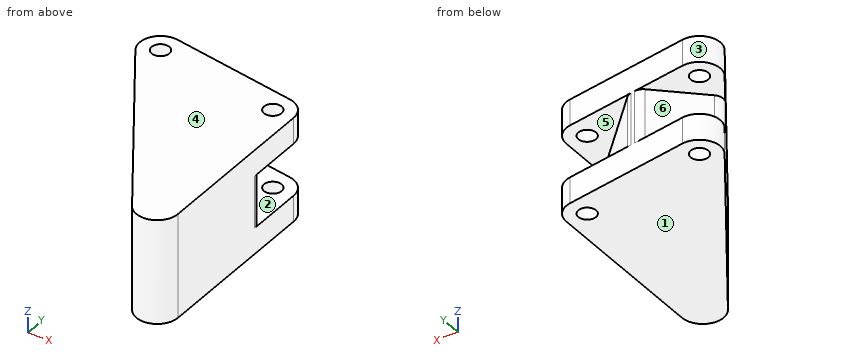
Autodesk Inventor part; units mm, degrees
ref_plane "YZ Plane" through (0, 0, 0) normal (1, 0, 0) x (0, 1, 0)
ref_plane "XZ Plane" through (0, 0, 0) normal (0, 1, 0) x (-1, 0, 0)
ref_plane "XY Plane" through (0, 0, 0) normal (0, 0, 1) x (1, 0, 0)
sketch "Sketch1" plane through (0, 0, 0) normal (0, 0, 1) x (1, 0, 0)
  line L0 (0, 0) -> (-24.2225, 3.8783) construction
  line L1 (-24.2225, 3.8783) -> (0, -32.7525) construction
  line L2 (0, -32.7525) -> (0, 0) construction
  line L3 (0.6324, 3.9497) -> (-23.5901, 7.828)
  line L4 (-27.559, 1.672) -> (-3.3365, -34.9588)
  line L5 (4, -32.7525) -> (4, 0)
  arc A0 (-23.5901, 7.828) -> (-27.559, 1.672) centre (-24.2225, 3.8783) ccw
  arc A1 (4, 0) -> (0.6324, 3.9497) centre (0, 0) ccw
  arc A2 (-3.3365, -34.9588) -> (4, -32.7525) centre (0, -32.7525) ccw
  dimension "d0" = 32.7525
  dimension "d6" = 24.531
  dimension "d14" = 43.9153
  dimension "d15" = 4
extrude "Extrusion1" add sketch "Sketch1" along normal mid plane 20
sketch "Sketch2" plane through (0, 0, 0) normal (0, 0, 1) x (1, 0, 0)
  arc A0 (-23.5901, 7.828) -> (-27.559, 1.672) centre (-24.2225, 3.8783) ccw construction
  line L0 (-3.3365, -34.9588) -> (-27.559, 1.672) construction
  arc A1 (-3.3365, -34.9588) -> (4, -32.7525) centre (0, -32.7525) ccw construction
  line L1 (4, 0) -> (4, -32.7525) construction
  arc A2 (4, 0) -> (0.6324, 3.9497) centre (0, 0) ccw construction
  line L2 (-23.5901, 7.828) -> (0.6324, 3.9497) construction
  arc A3 (4, 0) -> (0.6324, 3.9497) centre (0, 0) ccw
  line L3 (4, 0) -> (4, -10.3073)
  arc A4 (-3.3365, -34.9588) -> (4, -32.7525) centre (0, -32.7525) ccw construction
  line L4 (-3.3365, -34.9588) -> (-7.3441, -28.8984) construction
  arc A5 (-23.5901, 7.828) -> (-27.559, 1.672) centre (-24.2225, 3.8783) ccw
  line L5 (-23.5901, 7.828) -> (-14.2736, 6.3363)
  line L6 (-24.408, -3.0932) -> (-14.2736, 6.3363)
  line L7 (-11.9287, 5.9609) -> (4, -10.3073)
  line L8 (-7.3441, -28.8984) -> (4, -26.0222) construction
  line L9 (-24.408, -3.0932) -> (-27.559, 1.672)
  line L10 (-7.3441, -28.8984) -> (-24.408, -3.0932) construction
  line L11 (4, -10.3073) -> (4, -26.0222) construction
  line L12 (4, -26.0222) -> (4, -32.7525) construction
  line L13 (-11.9287, 5.9609) -> (0.6324, 3.9497)
  line L14 (-14.2736, 6.3363) -> (-11.9287, 5.9609) construction
extrude "Extrusion2" cut sketch "Sketch2" along normal mid plane 10
fillet "Fillet1" radius 2 4 edges at (4, -10.3073, 0) (-11.9287, 5.9609, 0) (-24.408, -3.0932, 0) (-14.2736, 6.3363, 0)
sketch "Sketch3" plane through (0, 0, 10) normal (0, 0, 1) x (1, 0, 0)
  arc A0 (-23.5901, 7.828) -> (-27.559, 1.672) centre (-24.2225, 3.8783) ccw construction
  arc A1 (-3.3365, -34.9588) -> (4, -32.7525) centre (0, -32.7525) ccw construction
  arc A2 (4, 0) -> (0.6324, 3.9497) centre (0, 0) ccw construction
hole "Hole1" at (-24.2225, 3.8783, 10) at (0, 0, 10) direction (0, 0, -1) diameter 3.4 end through all
equation "\"d0\" = LengthI"
equation "\"d6\" = LengthG"
equation "\"d14\" = LengthH"
properties part number "GHI"
Verification items for the finished model (mm, model axes). Face numbers are marked on the shaded views. A direction names the side the tool comes from. Round coordinates to 2 decimals unless told otherwise and drop trailing zeros. Order: outer loops, then holes, each group sorted by start corner. A loop starts at its lowest first (then second) coordinate and runs counter-clockwise, first axis right, second up.
1) Material ranges on line 1 (X direction, y = 1, z = 6.75); line 2 (Y direction, x = -24, z = 8.5); line 3 (X direction, y = 0, z = 8.9), recorded low to high.
Geometry says:
line 1: x = -27.11 to -1.37, 1.37 to 3.87
line 2: y = -3.71 to 2.19, 5.56 to 7.87
line 3: x = -26.45 to -1.7, 1.7 to 4
2) Depth check by flat-ended pin: pin 1 (2 mm diameter, centred on x = -20.5, z = 5, fed in from -Y); pin 2 (10 mm diameter, centred on y = -29.5, z = 2.5, fed in from -X); pin 3 (8 mm diameter, centred on y = -10, z = 2.5, fed in from -X). Enter the tip coordinate at first touch or a pass-through.
Geometry says:
pin 1: stops at y = -10.52
pin 2: stops at x = -10.25
pin 3: stops at x = -22.49
3) Draft check along Z on the marked faces 1, 2 and 3. Enter one of: +Z half, -Z half, draft (parallel to the pull), parting line (faces both ways), or undercut.
Geometry says:
face 1: -Z half
face 2: undercut
face 3: draft
4) Cross-section at B-B, the plane x = -21.5. Record the cut outline in (y, z).
Geometry says:
outline: (-7.49, -10) - (7.49, -10) - (7.49, -5) - (-0.39, -5) - (-0.39, 5) - (7.49, 5) - (7.49, 10) - (-7.49, 10) - close
5) Cross-section at D-D, the plane x = 0. Record the cut outline in (y, z), plus the area to 3 significant figures.
Geometry says:
outline: (-36.75, -10) - (-1.7, -10) - (-1.7, -5) - (-6.22, -5) - (-6.22, 5) - (-1.7, 5) - (-1.7, 10) - (-36.75, 10) - close; (1.7, -10) - (4.05, -10) - (4.05, -5) - (1.7, -5) - close; (1.7, 5) - (4.05, 5) - (4.05, 10) - (1.7, 10) - close
area: 679 mm2
6) Cross-section at A-A, the plane z = -6.5. Record the cut outline in (x, y), plus the area to 3 significant figures.
Geometry says:
outline: (-27.56, 1.67) - (-3.34, -34.96) arc R4 ccw to (4, -32.75) - (4, 0) arc R4 ccw to (0.63, 3.95) - (-23.59, 7.83) arc R4 ccw to start; hole circle Ø3.4 at (-24.22, 3.88); hole circle Ø3.4 at (0, 0)
area: 834 mm2
7) Tool access check on the marked faces 4, 5 and 6. Record the directions out of +Z, -Z, +X, -X, +Y, -Y that give a thin tool (end or side, any length) a straight path to the whole face; none if there is none.
Geometry says:
face 4: +Z, +X, -X, +Y, -Y
face 5: +X, +Y
face 6: -X, +Y
8) Cross-section at C-C, the plane y = -4. Record the cut outline in (x, z).
Geometry says:
outline: (-23.81, -10) - (4, -10) - (4, -5) - (-2.18, -5) - (-2.18, 5) - (4, 5) - (4, 10) - (-23.81, 10) - (-23.81, 5) - (-23.71, 5) - (-23.71, -5) - (-23.81, -5) - close
